```python
from build123d import *

# Parameters (mm, degrees)
F0_R     = 1.6
F1_DEPTH = 4
F2_DEPTH = 10
F3_DEPTH = 18
F4_R     = 1.75
F5_DEPTH = 23
F6_R     = 1


with BuildPart() as f1:
    # F0 (on Top) → F1 (new body)
    with BuildSketch(Plane.XY):
        Polygon((14, 0), (0, 0), (0, -18.75), (14, -18.75), (14, -16.875), (14, -1.875), align=None)
        with Locations((4.2, -14.55)):
            Circle(F0_R, mode=Mode.SUBTRACT)
    extrude(amount=F1_DEPTH)

    # F0 (on Top) → F2 (join)
    with BuildSketch(Plane.XY):
        Polygon((0, 3.8), (0, 0), (14, 0), (14, 2.125), (14, 3.8), align=None)
        Polygon((14, -18.75), (0, -18.75), (0, -22.55), (14, -22.55), (14, -20.875), align=None)
    extrude(amount=F2_DEPTH)

    # F0 (on Top) → F3 (join)
    with BuildSketch(Plane.XY):
        Polygon((14, 2.125), (14, 0), (14, -1.875), (28.4, -1.875), (28.4, 2.125), align=None)
        Polygon((14, -16.875), (14, -18.75), (14, -20.875), (28.4, -20.875), (28.4, -16.875), align=None)
    extrude(amount=F3_DEPTH)

    # F4 (on face) → F5 (cut, through all)
    with BuildSketch(Plane.XZ.offset(20.875)):
        with Locations((21.2, 13.5)):
            Circle(F4_R)
    extrude(amount=-F5_DEPTH, mode=Mode.SUBTRACT)

    # F6
    f6_edges = [f1.edges().sort_by_distance(p)[0] for p in [
        (0, -9.375, 4),
    ]]
    fillet(f6_edges, radius=F6_R)


solid = f1.part
```
Read the model definition and answer for the solid it produces. Units are mm, in the model's axes. A direction names the side the tool comes from. Round coordinates to 2 decimals unless told otherwise and drop trailing zeros. Write each loop counter-clockwise with the first axis right and the second up, starting at its lowest first coordinate (ties: lowest second). Pieces come first, ordered by that corner, then holes. Notation, with made-up numbers: (-12.5, 64.5) - (35.5, 64.5) arc R15 ccw to (35.5, 71.5) - close; hole circle Ø7 at (-15.75, 65.5). An arc over 180 degrees is marked (long way). One line per item, written item: value.
Q1. Find section D-D (z = 10.75). Determine the outline of the cut face in (x, y) (3 decimals).
The answers:
outline: (14, -20.875) - (28.4, -20.875) - (28.4, -16.875) - (14, -16.875) - close; (14, -1.875) - (28.4, -1.875) - (28.4, 2.125) - (14, 2.125) - close
Q2. Straight lines are drawn through the part: line 1 (Z direction, x = 21.2, y = -0.5); line 2 (Y direction, x = 16.5, z = 4.5) (3 decimals); line 3 (Y direction, x = 4.2, z = 2.5). For each, find the intervals that lie inside material, in ascending order. Write a range as from..to.
The answers:
line 1: z = 0..11.75, 15.25..18
line 2: y = -20.875..-16.875, -1.875..2.125
line 3: y = -22.55..-16.15, -12.95..3.8
Q3. For a pull along Y with two mould halves and no side action, classify faces 5 (the flat face through (14, 3, 5)), 6 (the cylindrical face through (0.301, -9.506, 3.715)), 7 (the flat face through (7, 3.8, 5)) as pulls with the +Y half, pulls with the -Y half, needs draft (parallel to the pull), parting line crosses it, or undercut.
The answers:
face 5: needs draft
face 6: undercut
face 7: pulls with the +Y half
Q4. Each of these flat-tipped pins is pushed along its axis until it touches: P1, Ø4, axis at x = 21.2, z = 13.5, coming from the -Y side (3 decimals); P2, Ø2, axis at x = 19.5, z = 2.5, coming from the +Y side (3 decimals); P3, Ø3, axis at x = 4.2, y = -14.55, coming from the +Z side; P4, Ø0.8, axis at y = -22, z = 3, coming from the +X side. Where does it stop, or does it pass through?
The answers:
P1: stops at y = -20.875
P2: stops at y = 2.125
P3: passes through
P4: stops at x = 14
Q5. Which of the six approach directions +Z, -Z, +X, -X, +Y, -Y give full straight-line access (tool end or side, diameter ignored) to faces 1 (the flat face through (14, -22, 5)), 2 (the flat face through (21, 2.125, 9)), 3 (the flat face through (14, -9, 2)), 4 (the flat face through (7, -18.75, 7))?
The answers:
face 1: +Z, -Z, +X, -Y
face 2: +Z, -Z, +X, +Y
face 3: +Z, -Z, +X
face 4: +Z, -X
Q6. Find section C-C (z = 13.5). Determine the outline of the cut face in (x, y) (3 decimals).
The answers:
outline: (14, -20.875) - (19.45, -20.875) - (19.45, -16.875) - (14, -16.875) - close; (14, -1.875) - (19.45, -1.875) - (19.45, 2.125) - (14, 2.125) - close; (22.95, -20.875) - (28.4, -20.875) - (28.4, -16.875) - (22.95, -16.875) - close; (22.95, -1.875) - (28.4, -1.875) - (28.4, 2.125) - (22.95, 2.125) - close
Q7. Find section A-A (x = 23.75). Determine the outline of the cut face in (y, z) (3 decimals), and give its area (3 significant figures).
The answers:
outline: (-20.875, 0) - (-16.875, 0) - (-16.875, 18) - (-20.875, 18) - close; (-1.875, 0) - (2.125, 0) - (2.125, 18) - (-1.875, 18) - close
area: 144 mm2
Q8. Find section B-B (y = -14.55). Determine the outline of the cut face in (x, z), and give its area (3 significant figures).
The answers:
outline: (0, 0) - (2.6, 0) - (2.6, 4) - (1, 4) arc R1 ccw to (0, 3) - close; (5.8, 0) - (14, 0) - (14, 4) - (5.8, 4) - close
area: 43.0 mm2
